Read the model definition and answer for the solid it produces. Units are mm, in the model's axes. Face numbers are marked on the shaded views. A direction names the side the tool comes from. Give positions to 0.01 mm unless a question says otherwise; leave off trailing zeros. Order: outer loops, then holes, each group sorted by start corner. A loop starts at its lowest first (then second) coordinate and runs counter-clockwise, first axis right, second up. Notation, with made-up numbers: (-2, 55.25) - (6, 55.25) arc R30 ccw to (6, 94.25) - close; hole circle Ø2 at (-12, -32). An arc over 180 degrees is marked (long way). Write each question's results on one line, items separated by ' | '. Start each with the question number.
Q1. Find section A-A on x = 0. Give the vertices of the cut face in (y, z) (3 decimals).
Q2. Find the intervals of material crossed by line 1 along Z through (x, y) = (-1.4, 0.55); line 2 along Y through (x, z) = (0.5, 2.5); line 3 along X through (y, z) = (0.55, 1.75), in increasing order. Write a range as from..to.
Q3. Flat-ended cylindrical pins translate along their axes: P1, Ø1.5, axis at y = 1, z = 2, coming from the +X side; P2, Ø1, axis at y = -1, z = 5, coming from the +X side; P3, Ø1.5, axis at y = 0, z = 5.5, coming from the +X side (3 decimals). Find the tip coordinate at first contact, or state that the pin passes through.
Q4. Find section C-C on z = 4.5. Give the vertices of the cut face in (x, y) (3 decimals).
Q5. Find section D-D on z = 0.5. Give the vertices of the cut face in (x, y) (3 decimals), and give its area (3 significant figures).
Q6. A tool of negligible diameter and unlimited length cuts with its end or side. For the marked faces 1, 2 and 3, from which of +Z, -Z, +X, -X, +Y, -Y can it reach the whole face along a straight path? Write none if from no direction.
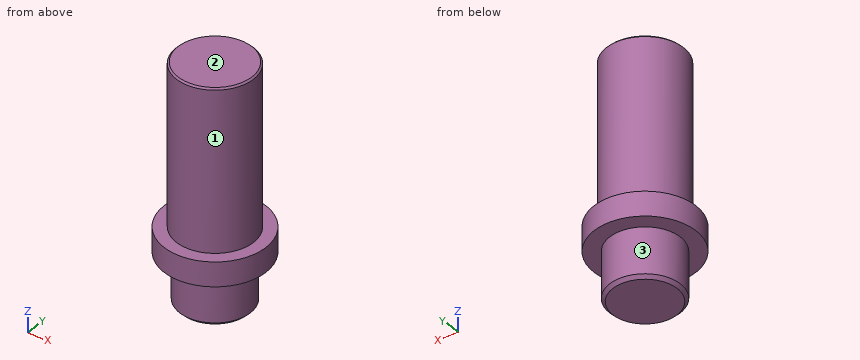
from build123d import *

# Parameters (mm, degrees)
CHAMFER_SIZE    = 0.1
CHAMFER001_SIZE = 0.05


with BuildPart() as part:
    # Sketch → Revolution (revolve)
    with BuildSketch(Plane.XZ):
        Polygon((0, 0), (1.105, 0), (1.105, 1.53), (1.59, 1.53), (1.59, 2.29), (1.205, 2.29), (1.205, 7.32), (0, 7.32), align=None)
    revolve(axis=Axis((0, 0, 0), (0, 0, 1)))

    # Chamfer
    chamfer_edges = [part.edges().sort_by_distance(p)[0] for p in [
        (-1.105, 0, 0),
    ]]
    chamfer(chamfer_edges, length=CHAMFER_SIZE)

    # Chamfer001
    chamfer001_edges = [part.edges().sort_by_distance(p)[0] for p in [
        (-1.205, 0, 7.32),
    ]]
    chamfer(chamfer001_edges, length=CHAMFER001_SIZE)


solid = part.part
Working result:
1) outline: (-1.59, 1.53) - (-1.105, 1.53) - (-1.105, 0.1) - (-1.005, 0) - (1.005, 0) - (1.105, 0.1) - (1.105, 1.53) - (1.59, 1.53) - (1.59, 2.29) - (1.205, 2.29) - (1.205, 7.27) - (1.155, 7.32) - (-1.155, 7.32) - (-1.205, 7.27) - (-1.205, 2.29) - (-1.59, 2.29) - close
2) line 1: 1.53..2.29 | line 2: -1.1..1.1 | line 3: -1.49..1.49
3) P1: x = 1.57 | P2: x = 1.1 | P3: x = 1.205
4) outline: circle Ø2.41 at (0, 0)
5) outline: circle Ø2.21 at (0, 0) | area: 3.84 mm²
6) face 1: +Z | face 2: +Z, +X, -X, +Y, -Y | face 3: -Z
